Work out the finished part from the listing and answer in its coordinate system (mm). A direction names the side the tool comes from. Give positions to 0.01 mm unless a question says otherwise; leave off trailing zeros. Order: outer loops, then holes, each group sorted by start corner. A loop starts at its lowest first (then second) coordinate and runs counter-clockwise, first axis right, second up. Notation, with made-up numbers: (4, 25.5) - (62, 25.5) arc R12 ccw to (62, 41.5) - close; hole circle Ø10 at (86, 74). An arc over 180 degrees is marked (long way). Put each result on its own line as item: value.
```python
from build123d import *

# Parameters (mm, degrees)
F1_DEPTH = 254
F2_R     = 50.8
F3_DEPTH = 148.336
F4_R     = 3.5438388493
F5_DEPTH = 89.916


with BuildPart() as f1:
    # F0 (on Right) → F1 (new body)
    with BuildSketch(Plane.YZ):
        with BuildLine():
            ThreePointArc((-25.4, -51.1953367017), (30.1206947131, -48.568160867), (57.15, 0))
            ThreePointArc((57.15, 0), (30.1206947131, 48.568160867), (-25.4, 51.1953367017))
            Line((-25.4, 51.1953367017), (-25.4, 43.9940905122))
            ThreePointArc((-25.4, 43.9940905122), (25.4, 43.9940905122), (50.8, 0))
            ThreePointArc((50.8, 0), (25.4, -43.9940905122), (-25.4, -43.9940905122))
            Line((-25.4, -43.9940905122), (-25.4, -51.1953367017))
        make_face()
    extrude(amount=F1_DEPTH)

    # F2 (on Top) → F3 (cut)
    with BuildSketch(Plane.XY):
        with Locations((177.8, 0)):
            Circle(F2_R)
    extrude(amount=F3_DEPTH, mode=Mode.SUBTRACT)

    # F4 (on Front) → F5 (cut)
    with BuildSketch(Plane.XZ):
        with Locations((127, -37.6440905122)):
            Circle(F4_R)
    extrude(amount=-F5_DEPTH, mode=Mode.SUBTRACT)


solid = f1.part
```
(1) Straight lines are drawn through the part: line 1 (Z direction, x = 127, y = 33.75); line 2 (Z direction, x = 224.5, y = 38.5); line 3 (Y direction, x = 238, z = 14.5). For each, find the intervals that lie inside material, in ascending order.
Geometry check:
line 1: z = -46.12 to -41.19, 37.97 to 46.12
line 2: z = -42.24 to -33.14, 33.14 to 42.24
line 3: y = 48.69 to 55.28
(2) Section A-A, the plane y = 0 is taken. Write down the section's boundary in (x, z), then the cut area to 3 significant figures.
Geometry check:
outline: (0, -57.15) - (254, -57.15) - (254, -50.8) - (0, -50.8) - close; (0, 50.8) - (127, 50.8) - (127, 57.15) - (0, 57.15) - close; (228.6, 50.8) - (254, 50.8) - (254, 57.15) - (228.6, 57.15) - close
area: 2,580 mm²
(3) Section C-C, the plane x = 233.5 is taken. Write down the section's boundary in (y, z), then the cut area to 3 significant figures.
Geometry check:
outline: (-25.4, -51.2) arc R57.15 ccw (long way) to (-25.4, 51.2) - (-25.4, 43.99) arc R50.8 cw (long way) to (-25.4, -43.99) - close
area: 1,410 mm²
(4) A tool of negligible diameter and unlimited length cuts with its end or side. For faces 3 (the face through (186.14, 50.11, 26.33)), 4 (the face through (254, 49.3, 13)), from which of +Z, -Z, +X, -X, +Y, -Y can it reach the whole face along a straight path? Write none if from no direction.
Geometry check:
face 3: +Z
face 4: +Z, -Z, +X, +Y, -Y
(5) Determine the mould class of faces 1 (the face through (128.635, 37.686, -40.788)), 2 (the face through (66, -25.4, 48)) for opening direction Z: pulls with the +Z half, pulls with the -Z half, needs draft (parallel to the pull), parting line crosses it, or undercut.
Geometry check:
face 1: undercut
face 2: needs draft
(6) Section D-D, the plane z = 4.5 is taken. Write down the section's boundary in (x, y), then the cut area to 3 significant figures.
Geometry check:
outline: (0, 50.6) - (173.3, 50.6) arc R50.8 cw to (182.3, 50.6) - (254, 50.6) - (254, 56.97) - (0, 56.97) - close
area: 1,620 mm²
(7) Given pin 1 (8 mm diameter, centred on x = 178.5, y = 36.5, fed in from +Z); pin 2 (5 mm diameter, centred on x = 119.5, y = -7, fed in from +Z); pin 3 (10 mm diameter, centred on x = 132.5, y = 48.5, fed in from -Z), each flat-ended and moving along its own axis, determine where each tip first touches the part or whether it passes through.
Geometry check:
pin 1: stops at z = -30.67
pin 2: stops at z = 56.97
pin 3: stops at z = -37.07
(8) Section B-B, the plane z = 32.5 is taken. Write down the section's boundary in (x, y), then the cut area to 3 significant figures.
Geometry check:
outline: (0, 39.04) - (145.3, 39.04) arc R50.8 cw to (158.54, 47.01) - (0, 47.01) - close; (197.06, 47.01) arc R50.8 cw to (210.3, 39.04) - (254, 39.04) - (254, 47.01) - close
area: 1,600 mm²
